Input: part model. Units: mm. Frame: model coordinates. Face numbers are marked on the shaded views. Round coordinates to 2 decimals unless told otherwise and drop trailing zeros. Loops run counter-clockwise (first coordinate to the right, second up) from the corner with the lowest first, then second, coordinate; pieces in that order, holes last.
(1) Line query: line 1 (Y direction, x = 43, z = 0.4); line 2 (X direction, y = -83.5, z = 0.25); line 3 (X direction, y = 39.5, z = 1.8). Output: solid intervals per line, ascending.
(2) Cut plane B-B, the plane y = 90. Output: boundary loops of the cut face in (x, z), and give its area (3 significant figures).
(3) Cut plane C-C, the plane x = 106.5. Output: boundary loops of the cut face in (y, z), and give its area (3 significant figures).
(4) First-contact query: pin 1 Ø1.5 at (y, z) = (98.5, 0.5) entering from -X. Flat tip, straight axial feed; report the tip coordinate or a pass-through.
(5) Cut plane A-A, the plane z = 0.6. Give the number of separate pieces and of enclosed holes in the cut face, and give its area (3 significant figures).
(6) Draft query along Z for the marked faces 1 and 2. Return one class per face: released by +Z, released by -Z, zero draft, split by the parting line, or undercut.
from build123d import *

# Parameters (mm, degrees)
F1_DEPTH = 4
F2_R     = 2.6
F3_DEPTH = 20
F4_R     = 2.6
F5_DEPTH = 4.001


# Not quite as in the source:
# - a feature names something its author has since deleted; it is built from what else it names


with BuildPart() as f1:
    # F0 (on Top) → F1 (new body)
    with BuildSketch(Plane.XY):
        Polygon((125.15, 79.85), (102.5, 102.5), (79.85, 125.15), (-79.9109665441, 125.15), (-102.530483272, 102.530483272), (-125.15, 79.9109665441), (-125.15, -79.85), (-102.5, -102.5), (-79.85, -125.15), (79.9109665441, -125.15), (102.530483272, -102.530483272), (125.15, -79.9109665441), align=None)
    extrude(amount=F1_DEPTH)

    # F2 (on face) → F3 (cut)
    with BuildSketch(Plane.XY.offset(4)):
        with Locations((-7.7781745931, 41.71930009)):
            Circle(F2_R)
        with Locations((-41.71930009, 7.7781745931)):
            Circle(F2_R)
        with Locations((7.7781745931, -41.71930009)):
            Circle(F2_R)
        with Locations((41.71930009, -7.7781745931)):
            Circle(F2_R)
        with Locations((41.71930009, 7.7781745931)):
            Circle(F2_R)
        with Locations((7.7781745931, 41.71930009)):
            Circle(F2_R)
        with Locations((-41.71930009, -7.7781745931)):
            Circle(F2_R)
        with Locations((-7.7781745931, -41.71930009)):
            Circle(F2_R)
    extrude(amount=-F3_DEPTH, mode=Mode.SUBTRACT)

    # F4 (on face) → F5 (cut, through all)
    with BuildSketch(Plane.XY.offset(4)):
        with Locations((-82.0243866176, 115.9655121146)):
            Circle(F4_R)
        with Locations((-115.9655121146, 82.0243866176)):
            Circle(F4_R)
        with Locations((82.0243866176, -115.9655121146)):
            Circle(F4_R)
        with Locations((115.9655121146, -82.0243866176)):
            Circle(F4_R)
        with Locations((82.0243866176, 115.9655121146)):
            Circle(F4_R)
        with Locations((115.9655121146, 82.0243866176)):
            Circle(F4_R)
        with Locations((-115.9655121146, -82.0243866176)):
            Circle(F4_R)
        with Locations((-82.0243866176, -115.9655121146)):
            Circle(F4_R)
    extrude(amount=-F5_DEPTH, mode=Mode.SUBTRACT)


solid = f1.part
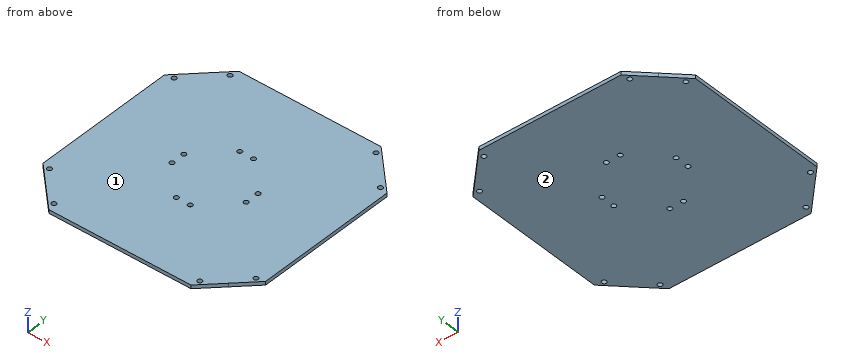
Reported:
1. line 1: y = -125.15 to -10.04, -5.52 to 5.52, 10.04 to 125.15
1. line 2: x = -121.5 to -118.11, -113.82 to 113.82, 118.11 to 121.56
1. line 3: x = -125.15 to -9.13, -6.42 to 6.42, 9.13 to 125.15
2. outline: (-115.06, 0) - (115, 0) - (115, 4) - (-115.06, 4) - close
2. area: 920 mm2
3. outline: (-98.56, 0) - (98.5, 0) - (98.5, 4) - (-98.56, 4) - close
3. area: 788 mm2
4. pin 1: stops at x = -107.31
5. separate pieces: 1
5. enclosed holes: 16
5. area: 58,200 mm2
6. face 1: released by +Z
6. face 2: released by -Z
